from build123d import *

# Parameters (mm, degrees)
BASE_W                   = 25.3
BASE_H                   = 9.5
RESSALTO_EXTRUS_O1_DEPTH = 3
ESBO_O4_W                = 8
ESBO_O4_H                = 3
CORTE_EXTRUS_O1_DEPTH    = 14.841423337
RESSALTO_EXTRUS_O2_DEPTH = 3
FILETE1_R                = 1
FILETE1_OF_ESPELHAR1_R   = 1


with BuildPart() as part:
    # Base → Ressalto-extrusão1 (new body)
    with BuildSketch(Plane.XY):
        Rectangle(BASE_W, BASE_H)
    extrude(amount=RESSALTO_EXTRUS_O1_DEPTH)

    # Esboço4 → Corte-extrusão1 (cut, through all)
    with BuildSketch(Plane.XY):
        Rectangle(ESBO_O4_W, ESBO_O4_H)
    extrude(amount=CORTE_EXTRUS_O1_DEPTH, mode=Mode.SUBTRACT)

    # Esboço2 → Ressalto-extrusão2 (add, through all)
    with BuildSketch(Plane.XY):
        with BuildLine():
            Line((-12.65, -3.35), (-15.85, -3.35))
            Line((-15.85, -3.35), (-15.85, -4.75))
            ThreePointArc((-15.85, -4.75), (-17.65, -2.95), (-15.85, -1.15))
            Line((-15.85, -1.15), (-15.85, 1.95))
            Line((-15.85, 1.95), (-12.65, 1.95))
            Line((-12.65, 1.95), (-12.65, -3.35))
        make_face()
    ressalto_extrus_o2 = extrude(amount=RESSALTO_EXTRUS_O2_DEPTH)

    # Filete1
    filete1_edges = [part.edges().sort_by_distance(p)[0] for p in [
        (-15.85, 1.95, 1.5),
    ]]
    fillet(filete1_edges, radius=FILETE1_R)

    # Espelhar1: Ressalto-extrusão2 across plane
    add(ressalto_extrus_o2.mirror(Plane(origin=(0, 0, 0), x_dir=(0, 0, 1), z_dir=(1, 0, 0))))

    # Filete1 of Espelhar1
    filete1_of_espelhar1_edges = [part.edges().sort_by_distance(p)[0] for p in [
        (15.85, 1.95, 1.5),
    ]]
    fillet(filete1_of_espelhar1_edges, radius=FILETE1_OF_ESPELHAR1_R)


solid = part.part
For this review, take the finished solid that the model builds, in its own axes (mm). A direction names the side the tool comes from. Round coordinates to 2 decimals unless told otherwise and drop trailing zeros. Order: outer loops, then holes, each group sorted by start corner. A loop starts at its lowest first (then second) coordinate and runs counter-clockwise, first axis right, second up. Notation, with made-up numbers: M 77,52.25 L 123,52.25 A13 ccw 123,70.25 Z; hole C 73,65 d9. An arc over 180 degrees is marked long. Use a Markdown table: item, result. Add a question column.
Item 1: Add section B-B, the plane y = 2.75. Give the boundary of the cut face in (x, z), then the cut area to 3 significant figures.
Item 2: To check wall thickness, follow line 1 along X through (y, z) = (-0.5, 1.35); line 2 along X through (y, z) = (2, 1.95); line 3 along Y through (x, z) = (14, 2.6). State the ranges of each line that lie inside material, in increasing order.
Item 3: Add section A-A, the plane z = 0.7. Give the boundary of the cut face in (x, y), then the cut area to 3 significant figures.
Item 4: Tool access review of faces 1 (the flat face through (-15.85, 0, 1)), 2 (the flat face through (-4, 0, 1)), 3 (the flat face through (12.65, 3, 1)): name each direction out of +Z, -Z, +X, -X, +Y, -Y from which nothing blocks a thin tool from reaching the whole face with its end or side.
Item 5: Insertion check: pin 1 (1.7 mm diameter, centred on y = 0.5, z = 1.5, fed in from -X); pin 2 (1.5 mm diameter, centred on y = -1, z = 2.5, fed in from +X); pin 3 (1.5 mm diameter, centred on x = 14, z = 1.5, fed in from -Y). Each pin has a flat end and moves straight along its axis. Give the tip position at first contact, or say it passes through.
Geometry results:
| question | item | result |
|---|---|---|
| 1 | outline | M -12.65,0 L 12.65,0 L 12.65,3 L -12.65,3 Z |
| 1 | area | 75.9 mm² |
| 2 | line 1 | x = -15.85 to -4, 4 to 15.85 |
| 2 | line 2 | x = -12.65 to 12.65 |
| 2 | line 3 | y = -3.35 to 1.95 |
| 3 | outline | M -15.85,-4.75 L -15.85,-3.35 L -12.65,-3.35 L -12.65,-4.75 L 12.65,-4.75 L 12.65,-3.35 L 15.85,-3.35 L 15.85,-4.75 A1.8 ccw 15.85,-1.15 L 15.85,0.95 A1 ccw 14.85,1.95 L 12.65,1.95 L 12.65,4.75 L -12.65,4.75 L -12.65,1.95 L -14.85,1.95 A1 ccw -15.85,0.95 L -15.85,-1.15 A1.8 ccw Z; hole M -4,-1.5 L 4,-1.5 L 4,1.5 L -4,1.5 Z |
| 3 | area | 260 mm² |
| 4 | face 1 | +Z, -Z, -X, +Y |
| 4 | face 2 | +Z, -Z |
| 4 | face 3 | +Z, -Z, +X, +Y |
| 5 | pin 1 | stops at x = -15.85 |
| 5 | pin 2 | stops at x = 17.19 |
| 5 | pin 3 | stops at y = -3.35 |
